Model file for the job. Use its own axes, mm. A direction names the side the tool comes from. Round coordinates to 2 decimals unless told otherwise and drop trailing zeros. Order: outer loops, then holes, each group sorted by start corner. A loop starts at its lowest first (then second) coordinate and runs counter-clockwise, first axis right, second up. Notation, with made-up numbers: (60.25, 48.25) -> (72.25, 48.25) arc R19 cw to (72.25, 69.25) -> close; hole circle Ø2 at (75, -2). An arc over 180 degrees is marked (long way). Put each result on its own line as item: value. Start each with the question number.
Q1. Cut at A-A, the plane z = 0. List the corners of the cut face in (x, y).
Q2. Cut at B-B, the plane x = 0. List the corners of the cut face in (y, z).
Q3. Flat gauge pin, fed straight in: P1, Ø6, axis at x = -3.5, y = 1.5, coming from the +Z side. Where does the tip first touch, or does it go through?
Q4. Cut at D-D, the plane y = 10. List the corners of the cut face in (x, z), and give its area (3 significant figures).
Q5. Cut at C-C, the plane x = -7. List the corners of the cut face in (y, z).
Q6. Probe L1, parallel to Z at x = 7, y = 6.75; L2, parallel to X at y = 8, z = -4; L3, parallel to X at y = 8, z = 1.75. List the from-to ranges inside material, lowest first.
Q7. 3-axis set-ups, long thin cutter, end or side, ignore diameter. For faces 5 (the face through (1.438, 6.451, -3.462)), 6 (the face through (6.47, 6.08, -2.05)): which of +Z, -Z, +X, -X, +Y, -Y reach the whole face in a straight line?
Q8. Pull direction Y, two halves, no side cores. Call faces 1 (the face through (2.4, 0, 2.4)), 2 (the face through (10.299, 2.958, -4.688)), 3 (the face through (7.906, 7.181, -6.236)), 4 (the face through (0, 6, 6)): released by +Y, released by -Y, zero draft, split by the parting line, or undercut.
from build123d import *

# Parameters (mm, degrees)
CROQUIS1_R              = 11.5
CROQUIS1_R_2            = 3
CROQUIS1_R_3            = 1
SALIENTE_EXTRUIR1_DEPTH = 12
CORTAR_EXTRUIR1_DEPTH   = 13
CORTAR_EXTRUIR2_START   = 10
CROQUIS3_R              = 1.5
CORTAR_EXTRUIR2_DEPTH   = 12
CORTAR_EXTRUIR3_START   = 10
CROQUIS4_R              = 5
CORTAR_EXTRUIR3_DEPTH   = 4


with BuildPart() as part:
    # Croquis1 → Saliente-Extruir1 (new body)
    with BuildSketch(Plane(origin=(0, 0, 0), x_dir=(1, 0, 0), z_dir=(0, 1, 0))):
        Circle(CROQUIS1_R)
        Circle(CROQUIS1_R_2, mode=Mode.SUBTRACT)
        with Locations((0, 7)):
            Circle(CROQUIS1_R_3, mode=Mode.SUBTRACT)
        with Locations((7, 0)):
            Circle(CROQUIS1_R_3, mode=Mode.SUBTRACT)
        with Locations((0, -7)):
            Circle(CROQUIS1_R_3, mode=Mode.SUBTRACT)
        with Locations((-7, 0)):
            Circle(CROQUIS1_R_3, mode=Mode.SUBTRACT)
    extrude(amount=SALIENTE_EXTRUIR1_DEPTH)

    # Croquis2 → Cortar-Extruir1 (cut, through all)
    with BuildSketch(Plane(origin=(0, 12, 0), x_dir=(1, 0, 0), z_dir=(0, 1, 0))):
        Polygon((7.866562941, 3.447145558), (5.038135816, 0.618718434), (2.828427125, 2.828427125), (5.656854249, 5.656854249), align=None)
        Polygon((5.656854249, 5.656854249), (3.447145558, 7.866562941), (0.618718434, 5.038135816), (2.828427125, 2.828427125), align=None)
    extrude(amount=-CORTAR_EXTRUIR1_DEPTH, mode=Mode.SUBTRACT)

    # Croquis3 → Cortar-Extruir2 (cut)
    with BuildSketch(Plane(origin=(2.828427125, 0, -2.828427125), x_dir=(-0.707106781, 0, -0.707106781), z_dir=(0.707106781, 0, -0.707106781)).offset(CORTAR_EXTRUIR2_START)):
        with Locations((0, 6)):
            Circle(CROQUIS3_R)
    extrude(amount=-CORTAR_EXTRUIR2_DEPTH, mode=Mode.SUBTRACT)

    # Croquis4 → Cortar-Extruir3 (cut)
    with BuildSketch(Plane(origin=(2.828427125, 0, -2.828427125), x_dir=(-0.707106781, 0, -0.707106781), z_dir=(0.707106781, 0, -0.707106781)).offset(CORTAR_EXTRUIR3_START)):
        with Locations((0, 6)):
            Circle(CROQUIS4_R)
    extrude(amount=-CORTAR_EXTRUIR3_DEPTH, mode=Mode.SUBTRACT)


solid = part.part
Ans:
1. outline: (-11.5, 0) -> (-8, 0) -> (-8, 12) -> (-11.5, 12) -> close; (-6, 0) -> (-3, 0) -> (-3, 12) -> (-6, 12) -> close; (3, 0) -> (6, 0) -> (6, 12) -> (3, 12) -> close; (8, 0) -> (11.5, 0) -> (11.5, 12) -> (8, 12) -> close
2. outline: (0, -11.5) -> (12, -11.5) -> (12, -8) -> (0, -8) -> close; (0, -6) -> (12, -6) -> (12, -3) -> (0, -3) -> close; (0, 3) -> (12, 3) -> (12, 6) -> (0, 6) -> close; (0, 8) -> (12, 8) -> (12, 11.5) -> (0, 11.5) -> close
3. P1: stops at z = 11.49
4. outline: (4.95, -9.19) -> (9.19, -4.95) -> (9.97, -5.73) arc R11.5 ccw (long way) to (5.73, -9.97) -> close; hole circle Ø2 at (-7, 0); hole circle Ø6 at (0, 0); hole circle Ø2 at (0, -7); hole circle Ø2 at (0, 7); hole (0.62, -5.04) -> (3.45, -7.87) -> (7.87, -3.45) -> (5.04, -0.62) -> close; hole circle Ø2 at (7, 0)
4. area: 341 mm^2
5. outline: (0, -9.12) -> (12, -9.12) -> (12, -1) -> (0, -1) -> close; (0, 1) -> (12, 1) -> (12, 9.12) -> (0, 9.12) -> close
6. L1: z = -5.16 to -4.31, -2.58 to -1, 1 to 9.12
6. L2: x = -10.78 to 1.66, 7.31 to 10.14, 10.48 to 10.78
6. L3: x = -11.37 to -2.44, 2.44 to 11.37
7. face 5: none
7. face 6: +Y, -Y
8. face 1: released by -Y
8. face 2: undercut
8. face 3: undercut
8. face 4: zero draft
